Design review of the part built by this model. Coordinates are the model's own, in mm. A direction names the side the tool comes from. Round coordinates to 2 decimals unless told otherwise and drop trailing zeros. Order: outer loops, then holes, each group sorted by start corner. A loop starts at its lowest first (then second) coordinate and runs counter-clockwise, first axis right, second up. Notation, with made-up numbers: (-19.75, 36) - (-5.75, 36) arc R7 cw to (-5.75, 44) - close; hole circle Ø5 at (50.25, -28). An arc over 180 degrees is marked (long way). Use CSV: the item, a comma, the result in double quotes.
from build123d import *

# Parameters (mm, degrees)
SKETCH_1_R          = 10
EXTRUDE_1_DEPTH     = 5
CUT_EXTRUDE_1_DEPTH = 3
SKETCH_4_R          = 1
CUT_EXTRUDE_3_DEPTH = 3
CUT_EXTRUDE_2_DEPTH = 5
SKETCH_5_R          = 2.75
CUT_EXTRUDE_4_DEPTH = 10


with BuildPart() as part:
    # 스케치1 → 보스-돌출1 (new body)
    with BuildSketch(Plane.XY):
        Circle(SKETCH_1_R)
    extrude(amount=EXTRUDE_1_DEPTH)

    # 스케치2 → 컷-돌출1 (cut)
    with BuildSketch(Plane.XY.offset(5)):
        Polygon((0, 4.618802154), (-4, 2.309401077), (-4, -2.309401077), (0, -4.618802154), (4, -2.309401077), (4, 2.309401077), align=None)
    extrude(amount=-CUT_EXTRUDE_1_DEPTH, mode=Mode.SUBTRACT)

    # 스케치4 → 컷-돌출3 (cut)
    with BuildSketch(Plane.XY.offset(5)):
        with Locations((0, 3.618802154)):
            Circle(SKETCH_4_R)
        with Locations((3.133974596, 1.809401077)):
            Circle(SKETCH_4_R)
        with Locations((3.133974596, -1.809401077)):
            Circle(SKETCH_4_R)
        with Locations((0, -3.618802154)):
            Circle(SKETCH_4_R)
        with Locations((-3.133974596, -1.809401077)):
            Circle(SKETCH_4_R)
        with Locations((-3.133974596, 1.809401077)):
            Circle(SKETCH_4_R)
    extrude(amount=-CUT_EXTRUDE_3_DEPTH, mode=Mode.SUBTRACT)

    # 스케치3 → 컷-돌출2 (cut)
    with BuildSketch(Plane.XY.offset(5)):
        with BuildLine():
            ThreePointArc((5.495834063, 6.549679989), (0, 8.55), (-5.495834063, 6.549679989))
            ThreePointArc((-5.495834063, 6.549679989), (-5.686882155, 4.365990307), (-3.503192473, 4.174942215))
            ThreePointArc((-3.503192473, 4.174942215), (0, 5.45), (3.503192473, 4.174942215))
            ThreePointArc((3.503192473, 4.174942215), (5.686882155, 4.365990307), (5.495834063, 6.549679989))
        make_face()
        with BuildLine():
            ThreePointArc((2.924272225, -8.034371908), (7.404517202, -4.275), (8.420106288, 1.484691919))
            ThreePointArc((8.420106288, 1.484691919), (6.624499596, 2.741989261), (5.367202254, 0.946382568))
            ThreePointArc((5.367202254, 0.946382568), (4.719838451, -2.725), (1.864009781, -5.121324783))
            ThreePointArc((1.864009781, -5.121324783), (0.937617441, -7.107979568), (2.924272225, -8.034371908))
        make_face()
        with BuildLine():
            ThreePointArc((-8.420106288, 1.484691919), (-7.404517202, -4.275), (-2.924272225, -8.034371908))
            ThreePointArc((-2.924272225, -8.034371908), (-0.937617441, -7.107979568), (-1.864009781, -5.121324783))
            ThreePointArc((-1.864009781, -5.121324783), (-4.719838451, -2.725), (-5.367202254, 0.946382568))
            ThreePointArc((-5.367202254, 0.946382568), (-6.624499596, 2.741989261), (-8.420106288, 1.484691919))
        make_face()
    extrude(amount=-CUT_EXTRUDE_2_DEPTH, mode=Mode.SUBTRACT)

    # 스케치5 → 컷-돌출4 (cut)
    with BuildSketch(Plane(origin=(0, 0, 0), x_dir=(-1, 0, 0), z_dir=(0, 0, -1))):
        Circle(SKETCH_5_R)
    extrude(amount=-CUT_EXTRUDE_4_DEPTH, mode=Mode.SUBTRACT)


solid = part.part
1) For faces 1 (the face through (-3.993, 2.322, 3.521)), 2 (the face through (4.746, -2.679, 2.535)), list the 3-axis set-ups (+Z, -Z, +X, -X, +Y, -Y) from which the entire face can be reached by the end or side of a thin tool; tool diameter is ignored.
Data:
face 1,"+Z"
face 2,"+Z, -Z"
2) We need section B-B (x = 2.5). Give the boundary of the cut face in (y, z), then the cut area to 3 significant figures.
Data:
outline,"(-9.68, 0) - (-8.12, 0) - (-8.12, 5) - (-9.68, 5) - close; (-4.84, 0) - (-1.15, 0) - (-1.15, 2) - (-3.18, 2) - (-3.18, 5) - (-4.84, 5) - close; (1.15, 0) - (4.84, 0) - (4.84, 5) - (3.18, 5) - (3.18, 2) - (1.15, 2) - close; (8.18, 0) - (9.68, 0) - (9.68, 5) - (8.18, 5) - close"
area,"40.1 mm2"
3) We need section A-A (y = 0). Give the boundary of the cut face in (x, z), then the cut area to 3 significant figures.
Data:
outline,"(-10, 0) - (-8.55, 0) - (-8.55, 5) - (-10, 5) - close; (-5.45, 0) - (-2.75, 0) - (-2.75, 2) - (-4, 2) - (-4, 5) - (-5.45, 5) - close; (2.75, 0) - (5.45, 0) - (5.45, 5) - (4, 5) - (4, 2) - (2.75, 2) - close; (8.55, 0) - (10, 0) - (10, 5) - (8.55, 5) - close"
area,"34.0 mm2"
4) The part is to be moulded in two halves that separate along Y. For faces 3 (the face through (1.984, -3.473, 3.521)), 4 (the face through (4.3, 0.1, 5)), 5 (the face through (-2.17, -9.76, 2.46)), say which applies: +Y half, -Y half, draft (parallel to the pull), parting line (faces both ways), or undercut.
Data:
face 3,"undercut"
face 4,"draft"
face 5,"parting line"
5) We need section C-C (z = 2.7). Give the boundary of the cut face in (x, y), then the cut area to 3 significant figures.
Data:
outline,"circle Ø20 at (0, 0); hole (-8.42, 1.48) arc R8.55 ccw to (-2.92, -8.03) arc R1.55 ccw to (-1.86, -5.12) arc R5.45 cw to (-5.37, 0.95) arc R1.55 ccw to start; hole (-5.5, 6.55) arc R1.55 ccw to (-3.5, 4.17) arc R5.45 cw to (3.5, 4.17) arc R1.55 ccw to (5.5, 6.55) arc R8.55 ccw to start; hole (-4, -1.31) arc R1 ccw to (-3.13, -2.81) - (-0.87, -4.12) arc R1 ccw to (0.87, -4.12) - (3.13, -2.81) arc R1 ccw to (4, -1.31) - (4, 1.31) arc R1 ccw to (3.13, 2.81) - (0.87, 4.12) arc R1 ccw to (-0.87, 4.12) - (-3.13, 2.81) arc R1 ccw to (-4, 1.31) - close; hole (1.86, -5.12) arc R1.55 ccw to (2.92, -8.03) arc R8.55 ccw to (8.42, 1.48) arc R1.55 ccw to (5.37, 0.95) arc R5.45 cw to start"
area,"144 mm2"
6) To check wall thickness, follow L1, parallel to Y at x = 0, z = 1.3; L2, parallel to X at y = -1.5, z = 1.85; L3, parallel to X at y = -6.5, z = 3.75. State the ranges of each line that lie inside material, in increasing order. Write a range as from..to.
Data:
L1,"y = -10..-2.75, 2.75..5.45, 8.55..10"
L2,"x = -9.89..-8.42, -5.24..-2.3, 2.3..5.24, 8.42..9.89"
L3,"x = -7.6..-5.55, -0.85..0.85, 5.55..7.6"
7) We need section D-D (x = 0). Give the boundary of the cut face in (y, z), then the cut area to 3 significant figures.
Data:
outline,"(-10, 0) - (-2.75, 0) - (-2.75, 2) - (-4.62, 2) - (-4.62, 5) - (-10, 5) - close; (2.75, 0) - (5.45, 0) - (5.45, 5) - (4.62, 5) - (4.62, 2) - (2.75, 2) - close; (8.55, 0) - (10, 0) - (10, 5) - (8.55, 5) - close"
area,"45.8 mm2"
8) Insertion check: pin 1 Ø3 at (x, z) = (-8, 3) entering from +Y; pin 2 Ø1 at (x, z) = (4, 3) entering from +Y; pin 3 Ø3.5 at (x, y) = (0, 0) entering from -Z. Each pin has a flat end and moves straight along its axis. Give the tip position at first contact, or say it passes through.
Data:
pin 1,"stops at y = 7.6"
pin 2,"stops at y = 9.37"
pin 3,"passes through"
